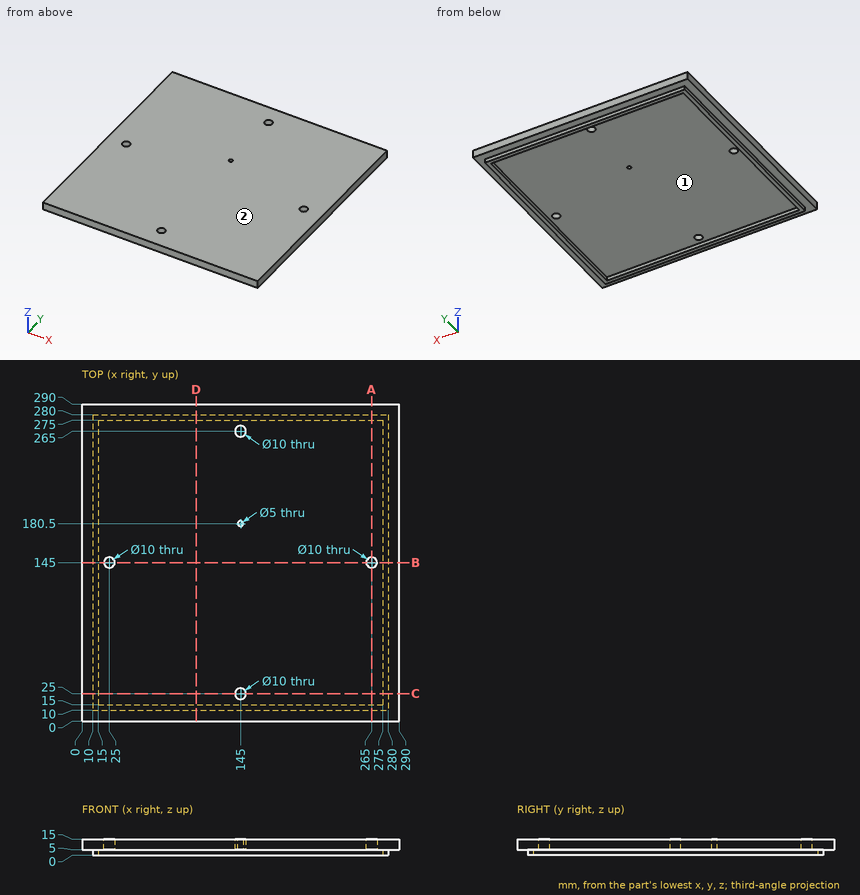
For this review, use the dimensioned drawing (mm, ordinates from the lowest corner) and the shaded views. Round coordinates to 2 decimals unless told otherwise and drop trailing zeros. Write each loop counter-clockwise with the first axis right and the second up, starting at its lowest first coordinate (ties: lowest second). Pieces come first, ordered by that corner, then holes. Notation, with made-up numbers: (-20.5, 36.5) -> (-10.5, 36.5) arc R23 cw to (-10.5, 56.5) -> close; hole circle Ø8 at (40, 80). An arc over 180 degrees is marked (long way). Use CSV: the item, a comma, the result in double quotes.
Q1. Consider section D-D (x = 104.5). Give the boundary of the cut face in (y, z), then the cut area to 3 significant figures.
Checks:
outline,"(0, 5) -> (10, 5) -> (10, 0) -> (15, 0) -> (15, 5) -> (275, 5) -> (275, 0) -> (280, 0) -> (280, 5) -> (290, 5) -> (290, 15) -> (0, 15) -> close"
area,"2,950 mm²"
Q2. For pin 1 Ø1.5 at (x, z) = (52, 2) entering from -Y; pin 2 Ø2.5 at (y, z) = (83.5, 1.5) entering from +X; pin 3 Ø2.5 at (x, z) = (169.5, 2.5) entering from +Y, all flat-tipped, find the tip position at first contact; note any pin that passes through.
Checks:
pin 1,"y = 10"
pin 2,"x = 280"
pin 3,"y = 280"
Q3. To check wall thickness, follow probe 1 along Y at (x, z) = (145, 7); probe 2 along X at (y, z) = (144.5, 10.5); probe 3 along Y at (x, z) = (140, 1). State the ranges of each line that lie inside material, in increasing order. Write a range as [from, to].
Checks:
probe 1,"[0, 20], [30, 178], [183, 260], [270, 290]"
probe 2,"[0, 20.03], [29.97, 260.03], [269.97, 290]"
probe 3,"[10, 15], [275, 280]"
Q4. Consider section A-A (x = 265). Give the boundary of the cut face in (y, z), then the cut area to 3 significant figures.
Checks:
outline,"(0, 5) -> (10, 5) -> (10, 0) -> (15, 0) -> (15, 5) -> (140, 5) -> (140, 15) -> (0, 15) -> close; (150, 5) -> (275, 5) -> (275, 0) -> (280, 0) -> (280, 5) -> (290, 5) -> (290, 15) -> (150, 15) -> close"
area,"2,850 mm²"
Q5. Consider section B-B (y = 145). Give the boundary of the cut face in (x, z), then the cut area to 3 significant figures.
Checks:
outline,"(0, 5) -> (10, 5) -> (10, 0) -> (15, 0) -> (15, 5) -> (20, 5) -> (20, 15) -> (0, 15) -> close; (30, 5) -> (260, 5) -> (260, 15) -> (30, 15) -> close; (270, 5) -> (275, 5) -> (275, 0) -> (280, 0) -> (280, 5) -> (290, 5) -> (290, 15) -> (270, 15) -> close"
area,"2,750 mm²"
Q6. Mouldability with a two-part tool opening along X and no side actions: class the marked faces 1 and 2 as released by +X, released by -X, zero draft, split by the parting line, or undercut.
Checks:
face 1,"undercut"
face 2,"zero draft"
